Verification items for this drawing (mm, ordinates from the low corner). Round coordinates to 2 decimals unless told otherwise and drop trailing zeros. Order: outer loops, then holes, each group sorted by start corner. A loop starts at its lowest first (then second) coordinate and runs counter-clockwise, first axis right, second up. Notation, with made-up numbers: (56, -3) - (78, -3) arc R25 cw to (78, 23) - close; hole circle Ø6 at (71, 74). An arc over 180 degrees is marked (long way). Use a Markdown table: item, result. Add a question column.
(1) Section check A-A on x = 56. Record the boundary of the cut face in (y, z) (1 decimal).
(2) Section check C-C on z = 10.5. Record the boundary of the cut face in (x, y) (1 decimal).
(3) Gauge pin test, flat end, axial feed: P1, Ø1.5, axis at x = 31.5, z = 104.5, coming from the -Y side. Record the tip position at first contact, or that the pin passes through.
(4) Section check B-B on y = 9. Record the boundary of the cut face in (x, z).
(5) Thickness scan on line 1 along Z through (x, y) = (95, 11); line 2 along Z through (x, y) = (106, 12.5); line 3 along Y through (x, z) = (111, 115.5). Record the ranges inside material, lowest first. Write a range as [from, to].
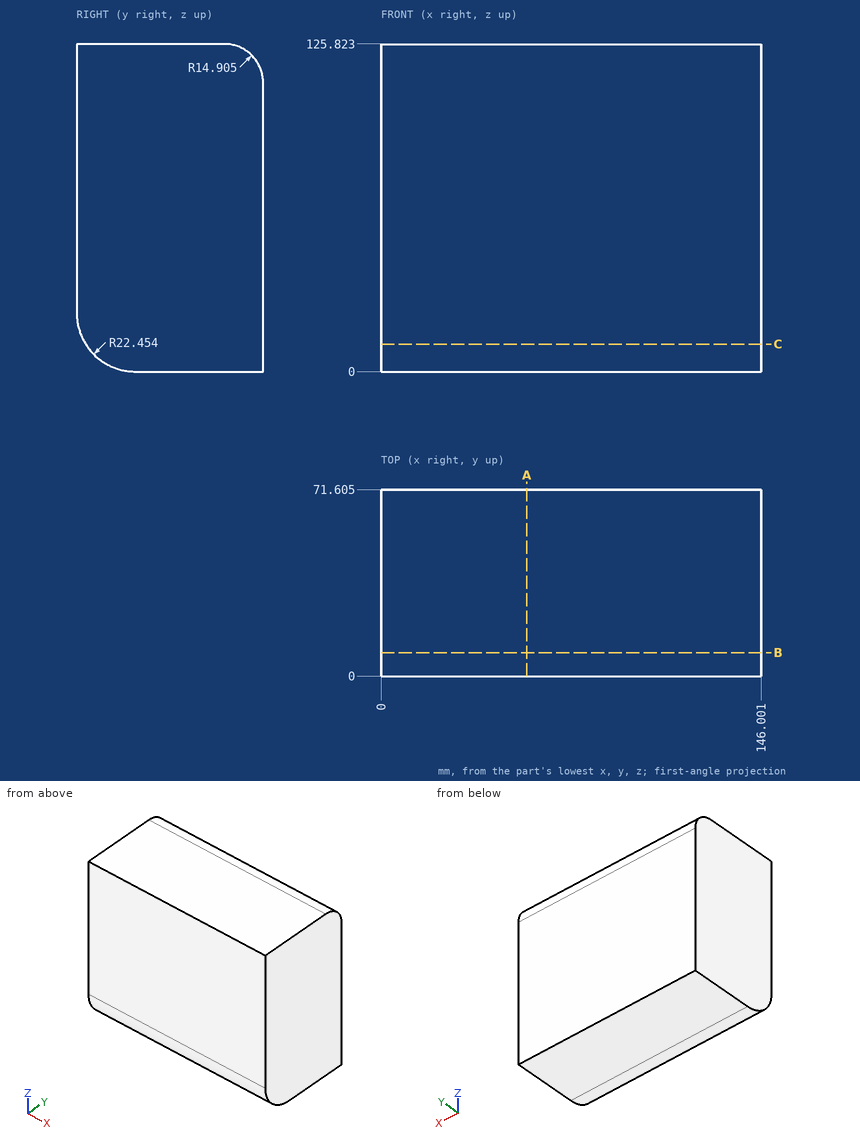
Check sheet entries:
| question | item | result |
|---|---|---|
| 1 | outline | (0, 22.5) arc R22.5 ccw to (22.5, 0) - (71.6, 0) - (71.6, 110.9) arc R14.9 ccw to (56.7, 125.8) - (0, 125.8) - close |
| 2 | outline | (0, 3.4) - (146, 3.4) - (146, 71.6) - (0, 71.6) - close |
| 3 | P1 | stops at y = 0 |
| 4 | outline | (0, 4.48) - (146, 4.48) - (146, 125.82) - (0, 125.82) - close |
| 5 | line 1 | z = [3.14, 125.82] |
| 5 | line 2 | z = [2.33, 125.82] |
| 5 | line 3 | y = [0, 70.88] |
